```python
from build123d import *

# Parameters (mm, degrees)
BOSS_EXTRUDE1_DEPTH            = 1.5
SKETCH2_W                      = 4.5
SKETCH2_H                      = 19.25
BOSS_EXTRUDE2_DEPTH            = 1.15
BOSS_EXTRUDE3_DEPTH            = 0.75
SKETCH4_W                      = 2.65
SKETCH4_H                      = 20
BOSS_EXTRUDE4_DEPTH            = 4.9
SKETCH5_W                      = 2.65
SKETCH5_H                      = 20
BOSS_EXTRUDE5_DEPTH            = 4.9
SKETCH6_W                      = 14.3
SKETCH6_H                      = 20
BOSS_EXTRUDE6_DEPTH            = 0.23
SKETCH7_W                      = 6.9
SKETCH7_H                      = 0.7
CUT_EXTRUDE1_DEPTH             = 22.99898649
CUT_EXTRUDE2_REACH             = 18.523
CUT_EXTRUDE3_REACH             = 18.523
SKETCH12_W                     = 6.5
SKETCH12_H                     = 0.23
CUT_EXTRUDE4_DEPTH             = 6.25
SKETCH13_W                     = 6.5
SKETCH13_H                     = 0.23
CUT_EXTRUDE5_DEPTH             = 6.249995
SKETCH14_W                     = 2.35
SKETCH14_H                     = 1.48
CUT_EXTRUDE6_DEPTH             = 22.99898649
SKETCH15_W                     = 2.35
SKETCH15_H                     = 1.48
CUT_EXTRUDE7_DEPTH             = 22.99898649
SKETCH16_W                     = 5.99999
SKETCH16_H                     = 5.99999
BOSS_EXTRUDE7_DEPTH            = 0.5
SKETCH17_W                     = 5.99999
SKETCH17_H                     = 5.99999
BOSS_EXTRUDE8_DEPTH            = 0.5
SKETCH18_W                     = 5.99999
SKETCH18_H                     = 5.99999
BOSS_EXTRUDE9_DEPTH            = 0.5
SKETCH19_W                     = 5.99999
SKETCH19_H                     = 5.99999
BOSS_EXTRUDE10_DEPTH           = 0.5
DRAFT1_ANGLE                   = 45
SKETCH20_W                     = 2.25
SKETCH20_H                     = 2
SKETCH21_W                     = 2.25
SKETCH21_H                     = 2
F_2_5_2_5_DIAMETER_HOLE1_D     = 2.5
F_2_5_2_5_DIAMETER_HOLE2_D     = 2.5
F_2_5_2_5_DIAMETER_HOLE2_DEPTH = 5.15
CHAMFER1_SIZE                  = 0.25


with BuildPart() as part:
    # Sketch1 → Boss-Extrude1 (new body)
    with BuildSketch(Plane.XY.offset(5.5)):
        with BuildLine():
            Line((1.993599736, -8.043101189), (2.25, -9))
            Line((2.25, -9), (2.25, 9))
            Line((2.25, 9), (1.993599736, 8.043101189))
            add(Edge.make_bspline(
                [(-1.993599736, 8.043101189), (-1.236487805, 9.490111472), (1.236487805, 9.490111472), (1.993599736, 8.043101189)],
                knots=[0, 0, 0, 0, 1, 1, 1, 1], degree=3))
            Line((-1.993599736, 8.043101189), (-2.25, 9))
            Line((-2.25, 9), (-2.25, -9))
            Line((-2.25, -9), (-1.993599736, -8.043101189))
            add(Edge.make_bspline(
                [(1.993599736, -8.043101189), (1.236487805, -9.490111472), (-1.236487805, -9.490111472), (-1.993599736, -8.043101189)],
                knots=[0, 0, 0, 0, 1, 1, 1, 1], degree=3))
        make_face()
    extrude(amount=-BOSS_EXTRUDE1_DEPTH)

    # Sketch2 → Boss-Extrude2 (add)
    with BuildSketch(Plane(origin=(0, 0, 4), x_dir=(-1, 0, 0), z_dir=(0, 0, -1))):
        with Locations((0, 0.375)):
            Rectangle(SKETCH2_W, SKETCH2_H)
    extrude(amount=BOSS_EXTRUDE2_DEPTH)

    # Sketch3 → Boss-Extrude3 (add)
    with BuildSketch(Plane.XZ.offset(9.25)):
        with BuildLine():
            Line((2.25, 2.85), (-2.25, 2.85))
            Line((-2.25, 2.85), (-2.25, 4))
            add(Edge.make_bspline(
                [(2.25, 4), (0.75, 4), (-0.75, 4), (-2.25, 4)],
                knots=[0, 0, 0, 0, 1, 1, 1, 1], degree=3))
            Line((2.25, 4), (2.25, 2.85))
        make_face()
    extrude(amount=BOSS_EXTRUDE3_DEPTH)

    # Sketch4 → Boss-Extrude4 (add)
    with BuildSketch(Plane(origin=(2.25, 0, 0), x_dir=(0, 0, -1), z_dir=(1, 0, 0))):
        with Locations((-4.175, 0)):
            Rectangle(SKETCH4_W, SKETCH4_H)
    extrude(amount=BOSS_EXTRUDE4_DEPTH)

    # Sketch5 → Boss-Extrude5 (add)
    with BuildSketch(Plane.ZY.offset(2.25)):
        with Locations((4.175, 0)):
            Rectangle(SKETCH5_W, SKETCH5_H)
    extrude(amount=BOSS_EXTRUDE5_DEPTH)

    # Sketch6 → Boss-Extrude6 (add)
    with BuildSketch(Plane.XY.offset(5.5)):
        Rectangle(SKETCH6_W, SKETCH6_H)
    extrude(amount=BOSS_EXTRUDE6_DEPTH)

    # Sketch7 → Cut-Extrude1 (cut, through all)
    with BuildSketch(Plane.XZ.offset(10)):
        with Locations((0, 3.2)):
            Rectangle(SKETCH7_W, SKETCH7_H)
    extrude(amount=-CUT_EXTRUDE1_DEPTH, mode=Mode.SUBTRACT)

    # Sketch9 → Cut-Extrude2 (cut, up to next)
    with BuildSketch(Plane(origin=(0, -3.75, 0), x_dir=(1, 0, 0), z_dir=(0, 1, 0)), mode=Mode.PRIVATE) as cut_extrude2_sk1:
        with BuildLine():
            Line((3.25, -4), (3.25, -3.55))
            Line((3.25, -3.55), (-3.25, -3.55))
            Line((-3.25, -3.55), (-3.25, -4))
            add(Edge.make_bspline(
                [(3.25, -4), (1.083333333, -4), (-1.083333333, -4), (-3.25, -4)],
                knots=[0, 0, 0, 0, 1, 1, 1, 1], degree=3))
        make_face()
    cut_extrude2_tool1 = extrude(cut_extrude2_sk1.sketch, amount=-CUT_EXTRUDE2_REACH, mode=Mode.PRIVATE) & part.part
    add(cut_extrude2_tool1.solids().sort_by_distance((0, -3.75, 3.775))[0], mode=Mode.SUBTRACT)

    # Sketch11 → Cut-Extrude3 (cut, up to next)
    with BuildSketch(Plane.XZ.offset(-3.75), mode=Mode.PRIVATE) as cut_extrude3_sk1:
        with BuildLine():
            Line((-3.25, 4), (-3.25, 3.55))
            Line((-3.25, 3.55), (3.25, 3.55))
            Line((3.25, 3.55), (3.25, 4))
            add(Edge.make_bspline(
                [(-3.25, 4), (-1.083333333, 4), (1.083333333, 4), (3.25, 4)],
                knots=[0, 0, 0, 0, 1, 1, 1, 1], degree=3))
        make_face()
    cut_extrude3_tool1 = extrude(cut_extrude3_sk1.sketch, amount=-CUT_EXTRUDE3_REACH, mode=Mode.PRIVATE) & part.part
    add(cut_extrude3_tool1.solids().sort_by_distance((0, 3.75, 3.775))[0], mode=Mode.SUBTRACT)

    # Sketch12 → Cut-Extrude4 (cut)
    with BuildSketch(Plane(origin=(0, 10, 0), x_dir=(-1, 0, 0), z_dir=(0, 1, 0))):
        with Locations((0, 5.615)):
            Rectangle(SKETCH12_W, SKETCH12_H)
    extrude(amount=-CUT_EXTRUDE4_DEPTH, mode=Mode.SUBTRACT)

    # Sketch13 → Cut-Extrude5 (cut)
    with BuildSketch(Plane.XZ.offset(10)):
        with Locations((0, 5.615)):
            Rectangle(SKETCH13_W, SKETCH13_H)
    extrude(amount=-CUT_EXTRUDE5_DEPTH, mode=Mode.SUBTRACT)

    # Sketch14 → Cut-Extrude6 (cut, through all)
    with BuildSketch(Plane(origin=(0, 10, 0), x_dir=(-1, 0, 0), z_dir=(0, 1, 0))):
        with Locations((5.975, 4.99)):
            Rectangle(SKETCH14_W, SKETCH14_H)
    extrude(amount=-CUT_EXTRUDE6_DEPTH, mode=Mode.SUBTRACT)

    # Sketch15 → Cut-Extrude7 (cut, through all)
    with BuildSketch(Plane(origin=(0, 10, 0), x_dir=(-1, 0, 0), z_dir=(0, 1, 0))):
        with Locations((-5.975, 4.99)):
            Rectangle(SKETCH15_W, SKETCH15_H)
    extrude(amount=-CUT_EXTRUDE7_DEPTH, mode=Mode.SUBTRACT)

    # Sketch16 → Boss-Extrude7 (add)
    with BuildSketch(Plane(origin=(0, 0, 4), x_dir=(-1, 0, 0), z_dir=(0, 0, -1))):
        with Locations((0, 7)):
            Rectangle(SKETCH16_W, SKETCH16_H)
    extrude(amount=BOSS_EXTRUDE7_DEPTH)

    # Sketch17 → Boss-Extrude8 (add)
    with BuildSketch(Plane.XY.offset(5.5)):
        with Locations((0, 7)):
            Rectangle(SKETCH17_W, SKETCH17_H)
    extrude(amount=BOSS_EXTRUDE8_DEPTH)

    # Sketch18 → Boss-Extrude9 (add)
    with BuildSketch(Plane(origin=(0, 0, 4), x_dir=(-1, 0, 0), z_dir=(0, 0, -1))):
        with Locations((0, -7)):
            Rectangle(SKETCH18_W, SKETCH18_H)
    extrude(amount=BOSS_EXTRUDE9_DEPTH)

    # Sketch19 → Boss-Extrude10 (add)
    with BuildSketch(Plane.XY.offset(5.5)):
        with Locations((0, -7)):
            Rectangle(SKETCH19_W, SKETCH19_H)
    extrude(amount=BOSS_EXTRUDE10_DEPTH)

    # Draft1
    draft1_faces = [part.faces().sort_by_distance(p)[0] for p in [
        (-3.45, 0, 3.2),
        (3.45, 0, 3.2),
    ]]
    draft(draft1_faces, Plane(origin=(3.45, 10, 3.55), x_dir=(-1, 0, 0), z_dir=(0, 0, -1)), DRAFT1_ANGLE)

    # Sketch20 → Revolve1 (revolve)
    with BuildSketch(Plane.XZ.offset(7), mode=Mode.PRIVATE) as revolve1_sk:
        with Locations((1.125, 7)):
            Rectangle(SKETCH20_W, SKETCH20_H)
    revolve(revolve1_sk.sketch.rotate(Axis((0, -7, 8.000025), (0, 0, -1)), 180), axis=Axis((0, -7, 8.000025), (0, 0, -1)))

    # Sketch21 → Revolve2 (revolve)
    with BuildSketch(Plane.XZ.offset(-7), mode=Mode.PRIVATE) as revolve2_sk:
        with Locations((1.125, 7)):
            Rectangle(SKETCH21_W, SKETCH21_H)
    revolve(revolve2_sk.sketch.rotate(Axis((0, 7, 8.000025), (0, 0, -1)), 180), axis=Axis((0, 7, 8.000025), (0, 0, -1)))

    # Ø2.5 (2.5) Diameter Hole1 (through all)
    with Locations(Plane(origin=(0, 0, 3.5), x_dir=(-1, 0, 0), z_dir=(0, 0, -1))):
        with Locations((0, -7)):
            Hole(F_2_5_2_5_DIAMETER_HOLE1_D / 2)

    # Ø2.5 (2.5) Diameter Hole2
    with Locations(Plane.XY.offset(8)):
        with Locations((0, 7)):
            Hole(F_2_5_2_5_DIAMETER_HOLE2_D / 2, depth=F_2_5_2_5_DIAMETER_HOLE2_DEPTH)

    # Chamfer1
    chamfer1_edges = [part.edges().sort_by_distance(p)[0] for p in [
        (2.25, -7, 8),
        (2.25, 7, 8),
        (-1.25, -7, 3.5),
        (-1.25, -7, 8),
        (1.25, 7, 3.5),
        (1.25, 7, 8),
    ]]
    chamfer(chamfer1_edges, length=CHAMFER1_SIZE)


solid = part.part
```
Model file for the job. Use its own axes, mm. A direction names the side the tool comes from. Round coordinates to 2 decimals unless told otherwise and drop trailing zeros. Order: outer loops, then holes, each group sorted by start corner. A loop starts at its lowest first (then second) coordinate and runs counter-clockwise, first axis right, second up. Notation, with made-up numbers: (41, 11.5) -> (56, 11.5) arc R23 cw to (56, 21.5) -> close; hole circle Ø4 at (77, -38). An arc over 180 degrees is marked (long way). Use one line per item in the form item = value.
Item 1: Cut at B-B, the plane z = 6.4. Write the cut outline in (x, y).
Returned:
outline = circle Ø4.5 at (0, -7); circle Ø4.5 at (0, 7); hole circle Ø2.5 at (0, -7); hole circle Ø2.5 at (0, 7)
Item 2: Tool access for faces 1 (the face through (1.4, -5.6, 3.5)), 2 (the face through (-4.8, 0, 5)), 3 (the face through (-2.25, 9.5, 4.7)), 4 (the face through (-2, 8.4, 6)): list every direction of +Z, -Z, +X, -X, +Y, -Y with a clear straight run to the whole face (end or side of a thin tool).
Returned:
face_1 = -Z, +Y, -Y
face_2 = +Z, -X, +Y, -Y
face_3 = +Y
face_4 = +Z
Item 3: Pull direction Z, two halves, no side cores. Call faces 5 (the face through (-2.25, -9.5, 4.7)), 6 (the face through (5, -10, 4)), 7 (the face through (0, 0, 5.73)), 8 (the face through (2.12, -8.51, 4.76)): released by +Z, released by -Z, zero draft, split by the parting line, or undercut.
Returned:
face_5 = undercut
face_6 = zero draft
face_7 = released by +Z
face_8 = undercut
Item 4: Cut at A-A, the plane y = -0.5. Write the cut outline in (x, z), and give its area (3 significant figures).
Returned:
outline = (-7.15, 2.85) -> (-4.15, 2.85) -> (-3.45, 3.55) -> (3.45, 3.55) -> (4.15, 2.85) -> (7.15, 2.85) -> (7.15, 4.25) -> (4.8, 4.25) -> (4.8, 5.73) -> (-4.8, 5.73) -> (-4.8, 4.25) -> (-7.15, 4.25) -> close
area = 28.9 mm^2
Item 5: Flat gauge pins, fed straight in: pin 1 Ø3 at (x, z) = (4.5, 7.5) entering from +Y; pin 2 Ø1.1 at (y, z) = (9.5, 5) entering from +X; pin 3 Ø6 at (x, y) = (4.5, 4.5) entering from +Z; pin 4 Ø0.6 at (x, y) = (-0.5, 9) entering from -Z. Where does each tip first touch, or does it go through?
Returned:
pin_1 = through
pin_2 = 4.8
pin_3 = 7.85
pin_4 = 3.5
Item 6: Drill centre lines: line 1 (Y direction, x = 0, z = 5.05); line 2 (X direction, y = -4.5, z = 3.75); line 3 (Y direction, x = 0, z = 6.2). Where is each one in solid material? Low to high.
Returned:
line_1 = -9.13 to -8.25, -5.75 to 5.75, 8.25 to 9.13
line_2 = -7.15 to -3.25, -3 to 3, 3.25 to 7.15
line_3 = -9.25 to -8.25, -5.75 to -4.75, 4.75 to 5.75, 8.25 to 9.25
Item 7: Cut at C-C, the plane x = 0. Give the number of separate pieces and of enclosed holes in the cut face, and give its area (3 significant figures).
Returned:
separate_pieces = 3
enclosed_holes = 0
area = 39.6 mm^2
